from build123d import *

# Parameters (mm, degrees)
CROQUIS1_R              = 5.000000002
SALIENTE_EXTRUIR1_DEPTH = 5
SALIENTE_EXTRUIR2_START = -5
CROQUIS2_R              = 4.26743785
SALIENTE_EXTRUIR2_DEPTH = 5


with BuildPart() as part:
    # Croquis1 → Saliente-Extruir1 (new body)
    with BuildSketch(Plane(origin=(0, 0, 0), x_dir=(-1, 0, 0), z_dir=(0, 0, -1))):
        with BuildLine():
            ThreePointArc((65.366552273, -43.922636472), (65.468760949, -38.737894565), (61.975170701, -34.905555535))
            add(Edge.make_bspline(
                [(48.815695063, -15.501711479), (50.328955685, -23.082906451), (52.395963263, -33.157522067), (61.975170701, -34.905555535)],
                knots=[0, 0, 0, 0, 1, 1, 1, 1], degree=3))
            ThreePointArc((48.815695063, -15.501711479), (45.934799024, -11.346655018), (41.137795802, -9.748901511))
            add(Edge.make_bspline(
                [(6.131666021, 7.899536167), (15.139972032, -1.656202419), (27.24511665, -10.665918482), (41.137795802, -9.748901511)],
                knots=[0, 0, 0, 0, 1, 1, 1, 1], degree=3))
            ThreePointArc((6.131666021, 7.899536167), (-4.598441285, 8.879996497), (-9.989918973, -0.448908775))
            add(Edge.make_bspline(
                [(-16.008618179, -18.26686517), (-15.797694107, -17.895825564), (-12.262638843, -11.871150313), (-10.546593735, -6.581162345), (-9.989918973, -0.448908775)],
                knots=[0, 0, 0, 0, 0.04039471, 0.656610986, 0.656610986, 0.656610986, 0.656610986], degree=3))
            ThreePointArc((-16.008618179, -18.26686517), (-11.761967136, -17.845761098), (-9.273993033, -21.312944188))
            add(Edge.make_bspline(
                [(-9e-09, -10.000000002), (-2.926729974, -11.686757621), (-7.513439547, -15.000663628), (-8.673577005, -19.940680978), (-9.273993033, -21.312944188)],
                knots=[0, 0, 0, 0, 0.464305351, 0.659664826, 0.659664826, 0.659664826, 0.659664826], degree=3))
            ThreePointArc((-9e-09, -10.000000002), (1.120487591, -9.937027099), (2.22686312, -9.748901509))
            add(Edge.make_bspline(
                [(35.978828296, -23.863233377), (28.058119493, -13.940958986), (14.675184196, -9.205569704), (2.22686312, -9.748901509)],
                knots=[0, 0, 0, 0, 1, 1, 1, 1], degree=3))
            ThreePointArc((35.978828296, -23.863233377), (38.199491242, -25.189759407), (40.727345447, -25.738365226))
            add(Edge.make_bspline(
                [(51.96076037, -40.419223819), (52.800264101, -33.487834784), (46.144416797, -28.374213166), (40.727345447, -25.738365226)],
                knots=[0, 0, 0, 0, 1, 1, 1, 1], degree=3))
            ThreePointArc((51.96076037, -40.419223819), (52.348210074, -43.621422867), (54.130381087, -46.309928491))
            add(Edge.make_bspline(
                [(60.429953363, -67.492405783), (57.103333259, -65.904114864), (55.916753892, -57.608938241), (57.449959784, -50.201518935), (54.130381087, -46.309928491)],
                knots=[0, 0, 0, 0, 0.425583063, 1, 1, 1, 1], degree=3))
            add(Edge.make_bspline(
                [(65.366552273, -43.922636472), (62.948824726, -48.37679887), (63.028170153, -56.438278724), (63.035847799, -64.90708051), (60.429953363, -67.492405783)],
                knots=[0, 0, 0, 0, 0.588886368, 1, 1, 1, 1], degree=3))
        make_face()
        with Locations(Location((-9e-09, -2e-09, 0), (0, 0, 180))):
            Circle(CROQUIS1_R, mode=Mode.SUBTRACT)
    extrude(amount=-SALIENTE_EXTRUIR1_DEPTH)

    # Croquis2 → Saliente-Extruir2 (add)
    with BuildSketch(Plane.XY.offset(5).offset(SALIENTE_EXTRUIR2_START)):
        with Locations((13.520610478, -21.733973978)):
            Circle(CROQUIS2_R)
    extrude(amount=SALIENTE_EXTRUIR2_DEPTH)


solid = part.part
Design review of the part built by this model. Coordinates are the model's own, in mm. A direction names the side the tool comes from. Coordinates: 2 decimals unless noted, no trailing zeros. Order: outer loops, then holes, each group sorted by start corner. A loop starts at its lowest first (then second) coordinate and runs counter-clockwise, first axis right, second up. Notation, with made-up numbers: M -10.75,85.5 L 30.25,85.5 A32 ccw 30.25,114.5 Z; hole C 10.5,0 d5. An arc over 180 degrees is marked long. Use a Markdown table: item, result.
(1) For P1, Ø1, axis at y = -12.5, z = 2.5, coming from the -X side; P2, Ø8, axis at x = 0, y = 0, coming from the -Z side; P3, Ø1, axis at y = -41.5, z = 1.5, coming from the +X side, all flat-tipped, find the tip position at first contact; note any pin that passes through.
Worked answers:
| item | result |
|---|---|
| P1 | stops at x = -47.58 |
| P2 | passes through |
| P3 | stops at x = -51.92 |
(2) For faces 4 (the cylindrical face through (-45.99, -11.39, 2.46)), 5 (the cylindrical face through (-1.1, -9.94, 2.46)), list the 3-axis set-ups (+Z, -Z, +X, -X, +Y, -Y) from which the entire face can be reached by the end or side of a thin tool; tool diameter is ignored.
Worked answers:
| item | result |
|---|---|
| face 4 | +Z, -Z, -X, +Y |
| face 5 | +Z, -Z, -Y |
(3) Add section A-A (y = -42). Give the boundary of the cut face in (x, z), then the cut area to 3 significant figures.
Worked answers:
| item | result |
|---|---|
| outline | M -65.87,0 L -51.96,0 L -51.96,5 L -65.87,5 Z |
| area | 69.5 mm2 |
(4) Draft analysis for pull direction X (two halves, no side actions). For faces 1 (the cylindrical face through (4.46, 8.95, 2.46)), 2 (the cylindrical face through (-38.17, -25.18, 2.46)), 3 (the cylindrical face through (-52.333, -43.579, 2.465)), state which applies: released by +X, released by -X, zero draft, split by the parting line, or undercut.
Worked answers:
| item | result |
|---|---|
| face 1 | split by the parting line |
| face 2 | undercut |
| face 3 | released by +X |
(5) Wall thickness on probe 1 along X at (y, z) = (0, 1.35); probe 2 along X at (y, z) = (3, 4.5); probe 3 along X at (y, z) = (-44, 3.25): over which ranges is each line inside the solid? List them lowest first.
Worked answers:
| item | result |
|---|---|
| probe 1 | x = -14.66 to -5, 5 to 10 |
| probe 2 | x = -11.12 to -4, 4 to 9.54 |
| probe 3 | x = -65.32 to -52.5 |
